from build123d import *

# Parameters (mm, degrees)
PAD_DEPTH            = 15
SKETCH001_R          = 4.25
HOLE_DEPTH           = 25
CHAMFER_SIZE         = 1
FILLET_R             = 10
FILLET001_R          = 1
FILLET002_R          = 10
PAD003_DEPTH         = 10
SKETCH010_R          = 4.25
HOLE005_DEPTH        = 25
POCKET002_DEPTH      = 6
POCKET002_DEPTH_BACK = 15
CHAMFER003_SIZE      = 1


with BuildPart() as part:
    # Sketch → Pad (new body, symmetric)
    with BuildSketch(Plane.XY):
        Polygon((-25, 0), (-17, 0), (-7.5, 4), (7.5, 4), (17, 0), (25, 0), (25, 4), (7.5, 8), (-7.5, 8), (-25, 4), align=None)
    extrude(amount=PAD_DEPTH, both=True)

    # Sketch001 → Hole (cut)
    with BuildSketch(Plane.XZ):
        Circle(SKETCH001_R)
    extrude(amount=-HOLE_DEPTH, mode=Mode.SUBTRACT)

    # Chamfer
    chamfer_edges = [part.edges().sort_by_distance(p)[0] for p in [
        (4.25, 4, 0),
        (4.25, 8, 0),
    ]]
    chamfer(chamfer_edges, length=CHAMFER_SIZE)

    # Fillet
    fillet_edges = [part.edges().sort_by_distance(p)[0] for p in [
        (-17, 0, 0),
        (17, 0, 0),
    ]]
    fillet(fillet_edges, radius=FILLET_R)

    # Fillet001
    fillet001_edges = [part.edges().sort_by_distance(p)[0] for p in [
        (25, 0, 0),
        (25, 4, 0),
        (-25, 0, 0),
        (-25, 4, 0),
    ]]
    fillet(fillet001_edges, radius=FILLET001_R)

    # Fillet002
    fillet002_edges = [part.edges().sort_by_distance(p)[0] for p in [
        (-7.5, 4, 0),
        (7.5, 4, 0),
        (7.5, 8, 0),
        (-7.5, 8, 0),
    ]]
    fillet(fillet002_edges, radius=FILLET002_R)

    # Sketch009 (on Face5 of Clone) → Pad003 (new body)
    with BuildSketch(Plane.XZ.offset(-4)):
        Polygon((10.75, -6.206515), (10.75, 6.206515), (0, 12.413031), (-10.75, 6.206515), (-10.75, -6.206515), (0, -12.413031), align=None)
    extrude(amount=-PAD003_DEPTH)

    # Sketch010 (on Face34 of Pad003) → Hole005 (cut)
    with BuildSketch(Plane.XZ.offset(-4)):
        Circle(SKETCH010_R)
    extrude(amount=-HOLE005_DEPTH, mode=Mode.SUBTRACT)

    # Sketch011 (on Face23 of Hole005) → Pocket002 (cut, two sides)
    with BuildSketch(Plane.XZ.offset(-4)) as pocket002_sk:
        Polygon((6.75, -3.897114), (6.75, 3.897114), (0, 7.794229), (-6.75, 3.897114), (-6.75, -3.897114), (0, -7.794229), align=None)
    extrude(amount=-POCKET002_DEPTH, mode=Mode.SUBTRACT)
    extrude(pocket002_sk.sketch, amount=POCKET002_DEPTH_BACK, mode=Mode.SUBTRACT)

    # Chamfer003
    chamfer003_edges = [part.edges().sort_by_distance(p)[0] for p in [
        (10.75, 14, 0),
        (5.375, 14, -9.309773),
        (5.375, 14, 9.309773),
        (-5.375, 14, -9.309773),
        (-5.375, 14, 9.309773),
        (-10.75, 14, 0),
        (4.25, 14, 0),
    ]]
    chamfer(chamfer003_edges, length=CHAMFER003_SIZE)


solid = part.part
Could you check a few things on this model? Use its own coordinates, in mm. A direction names the side the tool comes from. Round coordinates to 2 decimals unless told otherwise and drop trailing zeros. Write each loop counter-clockwise with the first axis right and the second up, starting at its lowest first coordinate (ties: lowest second). Pieces come first, ordered by that corner, then holes. Notation, with made-up numbers: (43, 53) - (75, 53) arc R7 ccw to (75, 63) - close; hole circle Ø7 at (-36.75, 85.5). An arc over 180 degrees is marked (long way). Put each result on its own line as item: value. Start each with the question number.
(1) Will these pins go through, and if not, where does the flat tip stop? pin 1 (10 mm diameter, centred on x = -5.5, z = 6.5, fed in from -Y); pin 2 (2 mm diameter, centred on y = 9, z = -5.5, fed in from +X); pin 3 (3 mm diameter, centred on x = 13, z = -6, fed in from -Y); pin 4 (7.5 mm diameter, centred on x = 0, z = 0, fed in from -Y).
(2) For faces 1 (the flat face through (-5.45, 10.088, -9.266)), 2 (the cylindrical face through (7.48, 7.94, 11.28)), 3 (the flat face through (2.9, 10, -3.4)), which set-ups out of +Z, -Z, +X, -X, +Y, -Y let a thin tool reach every point of the face, with its end or its side?
(3) Thinking about a two-plate mould opening in X: for faces 4 (the cylindrical face through (7.43, 3.81, 0.21)), 5 (the cylindrical face through (-7.509, 7.935, 11.171)), 6 (the flat face through (21, 0, 0)), which applies, released by +X, released by -X, zero draft, split by the parting line, or undercut?
(4) I want a section at C-C, the plane z = -10.75. Please give me the cut outline in (x, y).
(5) I want a section at B-B, the plane y = 11.25. Please give me the cut outline in (x, z), plus the area to 3 significant figures.
(6) I want a section at D-D, the plane x = -12. Please give me the cut outline in (y, z), plus the area to 3 significant figures.
(7) I need wall thicknesses on probe 1 along Z at (x, y) = (0, 11.1); probe 2 along X at (y, z) = (0.75, -5); probe 3 along Z at (x, y) = (2, 5.5). Which ranges of each line are inside material? Lowest first, please.
Here are the results:
1. pin 1: stops at y = 2.74
1. pin 2: stops at x = 10.75
1. pin 3: stops at y = 1.05
1. pin 4: passes through
2. face 1: -Z, -X, +Y
2. face 2: +Z, +X, +Y
2. face 3: -Y
3. face 4: undercut
3. face 5: released by -X
3. face 6: zero draft
4. outline: (-25, 1) arc R1 ccw to (-24, 0) - (-19.02, 0) arc R10 ccw to (-15.14, 0.78) - (-9.36, 3.22) arc R10 cw to (-5.48, 4) - (5.48, 4) arc R10 cw to (9.36, 3.22) - (15.14, 0.78) arc R10 ccw to (19.02, 0) - (24, 0) arc R1 ccw to (25, 1) - (25, 3.2) arc R1 ccw to (24.22, 4.18) - (8.6, 7.75) arc R10 ccw to (6.37, 8) - (2.88, 8) - (2.88, 13) - (0.88, 14) - (-0.88, 14) - (-2.88, 13) - (-2.88, 8) - (-6.37, 8) arc R10 ccw to (-8.6, 7.75) - (-24.22, 4.18) arc R1 ccw to (-25, 3.2) - close
5. outline: (-10.75, -6.21) - (0, -12.41) - (10.75, -6.21) - (10.75, 6.21) - (0, 12.41) - (-10.75, 6.21) - close; hole circle Ø8.5 at (0, 0)
5. area: 344 mm^2
6. outline: (2.11, -15) - (6.97, -15) - (6.97, 15) - (2.11, 15) - close
6. area: 146 mm^2
7. probe 1: z = -12.41 to -4.25, 4.25 to 12.41
7. probe 2: x = -24.97 to -15.22, 15.22 to 24.97
7. probe 3: z = -15 to -6.64, 6.64 to 15
